The model under review builds one solid part; all positions refer to its coordinate system, in mm. Face numbers are marked on the shaded views. A direction names the side the tool comes from. Round coordinates to 2 decimals unless told otherwise and drop trailing zeros. Order: outer loops, then holes, each group sorted by start corner. A loop starts at its lowest first (then second) coordinate and runs counter-clockwise, first axis right, second up. Notation, with made-up numbers: (86, 17) -> (104, 17) arc R6 cw to (104, 27) -> close; hole circle Ø11 at (20, 40). An arc over 180 degrees is marked (long way). Use a Markdown table: item, result. Add a question column.
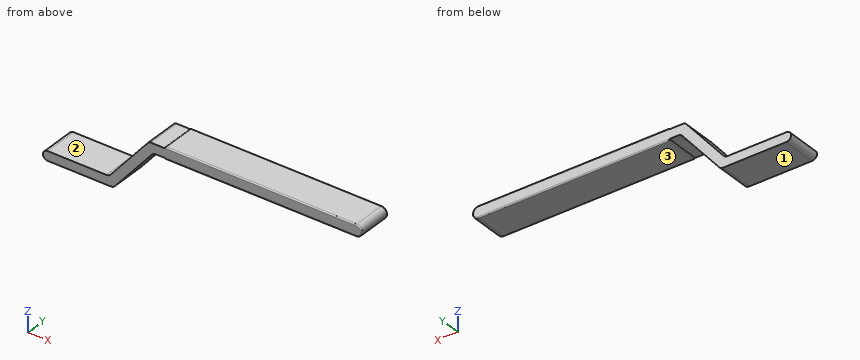
```python
from build123d import *

# Parameters (mm, degrees)
F1_DEPTH = 30
F2_R     = 0.99999


# Not quite as in the source:
# - a fillet or chamfer is up to 0.001 mm smaller than in the source, because OpenCascade refuses the exact size


with BuildPart() as f1:
    # F0 (on Front) → F1 (new body)
    with BuildSketch(Plane.XZ):
        with BuildLine():
            Line((-63.6692684564, 20.8099257126), (-114.3268977837, 20.8099257126))
            ThreePointArc((-114.3268977837, 20.8099257126), (-118.3668602392, 16.7699632572), (-114.3268977837, 12.7300008017))
            Line((-114.3268977837, 12.7300008017), (-59.988057444, 12.7300008017))
            ThreePointArc((-59.988057444, 12.7300008017), (-57.8669121635, 13.2022262159), (-56.1464303666, 14.5297037219))
            Line((-56.1464303666, 14.5297037219), (-24.0653757294, 53.0397061037))
            ThreePointArc((-24.0653757294, 53.0397061037), (-22.8610384715, 53.9689403579), (-21.3762367753, 54.2994981479))
            Line((-21.3762367753, 54.2994981479), (-13.1770761366, 54.2994981479))
            Line((-13.1770761366, 54.2994981479), (-13.1770761366, 62.2994981479))
            Line((-13.1770761366, 62.2994981479), (-25.1240298515, 62.2994981479))
            ThreePointArc((-25.1240298515, 62.2994981479), (-26.6088315478, 61.9689403579), (-27.8131688056, 61.0397061037))
            Line((-27.8131688056, 61.0397061037), (-59.8276413791, 22.6096286329))
            ThreePointArc((-59.8276413791, 22.6096286329), (-61.548123176, 21.2821511269), (-63.6692684564, 20.8099257126))
        make_face()
        with BuildLine():
            Line((-13.1770761366, 63.2994981479), (-13.1770761366, 62.2994981479))
            Line((-13.1770761366, 62.2994981479), (-13.1770761366, 54.2994981479))
            Line((-13.1770761366, 54.2994981479), (-13.1770761366, 53.2994981479))
            Line((-13.1770761366, 53.2994981479), (151.8229238634, 53.2994981479))
            ThreePointArc((151.8229238634, 53.2994981479), (156.8229238634, 58.2994981479), (151.8229238634, 63.2994981479))
            Line((151.8229238634, 63.2994981479), (-13.1770761366, 63.2994981479))
        make_face()
    extrude(amount=F1_DEPTH)

    # F2 (radius 1 in the source; OpenCascade refuses exactly that, so slightly less here)
    f2_edges = [f1.edges().sort_by_distance(p)[0] for p in [
        (69.322924, 0, 63.299498),
        (69.322924, -30, 53.299498),
        (151.822924, -15, 63.299498),
        (151.822924, -15, 53.299498),
        (-13.177076, -15, 53.299498),
        (-13.177076, -15, 63.299498),
    ]]
    fillet(f2_edges, radius=F2_R)


solid = f1.part
```
Q1. Add section A-A, the plane x = 133.5. Give the boundary of the cut face in (y, z).
Q2. For pin 1 (6 mm diameter, centred on y = -9, z = 49, fed in from -X); pin 2 (9.5 mm diameter, centred on x = -20, y = -20.5, fed in from +Z); pin 3 (2.5 mm diameter, centred on x = -18.5, y = -15, fed in from -Z), all flat-tipped, find the tip position at first contact; note any pin that passes through.
Q3. Add section D-D, the plane x = -95. Give the boundary of the cut face in (y, z), then the cut area to 3 significant figures.
Q4. For the marked faces 1, 2 and 3, list the 3-axis set-ups (+Z, -Z, +X, -X, +Y, -Y) from which the entire face can be reached by the end or side of a thin tool; tool diameter is ignored.
Q5. Add section C-C, the plane z = 45. Give the boundary of the cut face in (x, y), then the cut area to 3 significant figures.
Q6. To check wall thickness, follow line 1 along Z through (x, y) = (92.5, -9.75); line 2 along Z through (x, y) = (-64, -21.25); line 3 along X through (y, z) = (-11, 54). State the ranges of each line that lie inside material, in increasing order.
Return value:
| question | item | result |
|---|---|---|
| 1 | outline | (-30, 54.3) arc R1 ccw to (-29, 53.3) -> (-1, 53.3) arc R1 ccw to (0, 54.3) -> (0, 62.3) arc R1 ccw to (-1, 63.3) -> (-29, 63.3) arc R1 ccw to (-30, 62.3) -> close |
| 2 | pin 1 | x = -40.34 |
| 2 | pin 2 | z = 62.3 |
| 2 | pin 3 | z = 54.3 |
| 3 | outline | (-30, 12.73) -> (0, 12.73) -> (0, 20.81) -> (-30, 20.81) -> close |
| 3 | area | 242 mm² |
| 4 | face 1 | -Z, +X, -X, +Y, -Y |
| 4 | face 2 | +Z, -X, +Y, -Y |
| 4 | face 3 | -Z, +X, +Y, -Y |
| 5 | outline | (-41.18, -30) -> (-30.76, -30) -> (-30.76, 0) -> (-41.18, 0) -> close |
| 5 | area | 312 mm² |
| 6 | line 1 | 53.3 to 63.3 |
| 6 | line 2 | 12.73 to 20.81 |
| 6 | line 3 | -33.68 to -22.79, -13.13 to 154.38 |
